```python
from build123d import *
from build123d.topology import SkipClean

# Parameters (mm, degrees)
SALIENTE_EXTRUIR3_DEPTH        = 342.9
SALIENTE_EXTRUIR3_DEPTH_BACK   = 342.9
CROQUIS3_R                     = 6.35
SALIENTE_EXTRUIR3_2_DEPTH      = 342.9
SALIENTE_EXTRUIR3_2_DEPTH_BACK = 342.9
CROQUIS4_W                     = 533.4
CROQUIS4_H                     = 165.1
SALIENTE_EXTRUIR4_DEPTH        = 555.498
VACIADO3_START                 = -265.43
VACIADO3_DEPTH                 = 530.86
VACIADO3_START_2               = -341.63
VACIADO3_2_OUTLINE_R           = 5.08
VACIADO3_2_DEPTH               = 683.26
REDONDEO5_R                    = 2.54
CROQUIS5_W                     = 152.4
CROQUIS5_H                     = 2.54
SALIENTE_EXTRUIR5_DEPTH        = 101.6
CORTAR_EXTRUIR2_DEPTH          = 676.270787465
CORTAR_EXTRUIR8_DEPTH          = 676.270787542


# Read off the part's stored shape, not the designer's step: Vaciado3
with BuildPart() as part:
    # Croquis3 → Saliente-Extruir3 (new, two sides: drawn at the far end of the back side and taken through both)
    with BuildSketch(Plane(origin=(0, 0, 0), x_dir=(0, 0, -1), z_dir=(1, 0, 0)).offset(-SALIENTE_EXTRUIR3_DEPTH_BACK)):
        Circle(CROQUIS3_R)
    extrude(amount=SALIENTE_EXTRUIR3_DEPTH + SALIENTE_EXTRUIR3_DEPTH_BACK)



with BuildPart() as body_2:
    # Croquis3 → Saliente-Extruir3 2 (new, two sides: drawn at the far end of the back side and taken through both)
    with BuildSketch(Plane(origin=(0, 0, 0), x_dir=(0, 0, -1), z_dir=(1, 0, 0)).offset(-SALIENTE_EXTRUIR3_2_DEPTH_BACK)):
        with Locations((165.1, 0)):
            Circle(CROQUIS3_R)
    extrude(amount=SALIENTE_EXTRUIR3_2_DEPTH + SALIENTE_EXTRUIR3_2_DEPTH_BACK)


with BuildPart() as part_1:
    add(part.part)

    add(body_2.part)  # Saliente-Extruir4 merges body 2
    # Croquis4 → Saliente-Extruir4 (add)
    with BuildSketch(Plane(origin=(0, 0, 0), x_dir=(1, 0, 0), z_dir=(0, 1, 0))):
        with Locations((0, 82.55)):
            Rectangle(CROQUIS4_W, CROQUIS4_H)
    extrude(amount=-SALIENTE_EXTRUIR4_DEPTH)

    # Vaciado3 outline → Vaciado3 (cut)
    with BuildSketch(Plane.YZ.offset(VACIADO3_START)):
        with BuildLine():
            Line((-554.228, -163.83), (-4.91868885, -163.83))
            ThreePointArc((-4.91868885, -163.83), (3.110851973, -169.116092628), (0, -160.02))
            Line((0, -160.02), (0, -5.08))
            ThreePointArc((0, -5.08), (3.110851973, 4.016092628), (-4.91868885, -1.27))
            Line((-4.91868885, -1.27), (-554.228, -1.27))
            Line((-554.228, -1.27), (-554.228, -163.83))
        make_face()
    extrude(amount=VACIADO3_DEPTH, mode=Mode.SUBTRACT)

    # Vaciado3 2 outline → Vaciado3 2 (cut)
    with BuildSketch(Plane.YZ.offset(VACIADO3_START_2)):
        with Locations((0, -165.1)):
            Circle(VACIADO3_2_OUTLINE_R)
        Circle(VACIADO3_2_OUTLINE_R)
    extrude(amount=VACIADO3_2_DEPTH, mode=Mode.SUBTRACT)

    # Redondeo5
    # the kernel refuses this fillet: 2.54 mm, written as the material it takes off along each edge
    with BuildSketch(Plane(origin=(-264.16, -552.958, -2.54), x_dir=(0, 0, 1), z_dir=(-1, 0, 0))) as redondeo5_piece_1_section:
        Polygon((0, 0), (REDONDEO5_R * 1.02, 0), (REDONDEO5_R * 1.02, -REDONDEO5_R * 1.02), (0, -REDONDEO5_R * 1.02), align=None)
    redondeo5_piece_1 = extrude(amount=REDONDEO5_R * 1.02, mode=Mode.PRIVATE)
    redondeo5_piece_1 = redondeo5_piece_1 - Plane(origin=(-264.16, -552.958, -2.54), x_dir=(0, 0.7071067811865475, -0.7071067811865475), z_dir=(-1, 0, 0)) * Sphere(REDONDEO5_R, mode=Mode.PRIVATE)
    add(redondeo5_piece_1, mode=Mode.SUBTRACT)
    with BuildSketch(Plane(origin=(-264.16, -552.958, -162.56), x_dir=(0, -1, 0), z_dir=(-1, 0, 0))) as redondeo5_piece_2_section:
        Polygon((0, 0), (REDONDEO5_R * 1.02, 0), (REDONDEO5_R * 1.02, -REDONDEO5_R * 1.02), (0, -REDONDEO5_R * 1.02), align=None)
    redondeo5_piece_2 = extrude(amount=REDONDEO5_R * 1.02, mode=Mode.PRIVATE)
    redondeo5_piece_2 = redondeo5_piece_2 - Plane(origin=(-264.16, -552.958, -162.56), x_dir=(0, 0.7071067811865475, 0.7071067811865475), z_dir=(-1, 0, 0)) * Sphere(REDONDEO5_R, mode=Mode.PRIVATE)
    add(redondeo5_piece_2, mode=Mode.SUBTRACT)
    with BuildSketch(Plane(origin=(264.16, -552.958, -2.54), x_dir=(1, 0, 0), z_dir=(0, 0, 1))) as redondeo5_piece_3_section:
        Polygon((0, 0), (REDONDEO5_R * 1.02, 0), (REDONDEO5_R * 1.02, -REDONDEO5_R * 1.02), (0, -REDONDEO5_R * 1.02), align=None)
    redondeo5_piece_3 = extrude(amount=REDONDEO5_R * 1.02, mode=Mode.PRIVATE)
    redondeo5_piece_3 = redondeo5_piece_3 - Plane(origin=(264.16, -552.958, -2.54), x_dir=(-0.7071067811865475, 0.7071067811865475, 0), z_dir=(0, 0, 1)) * Sphere(REDONDEO5_R, mode=Mode.PRIVATE)
    add(redondeo5_piece_3, mode=Mode.SUBTRACT)
    with BuildSketch(Plane(origin=(264.16, -552.958, -162.56), x_dir=(1, 0, 0), z_dir=(0, -1, 0))) as redondeo5_piece_4_section:
        Polygon((0, 0), (REDONDEO5_R * 1.02, 0), (REDONDEO5_R * 1.02, -REDONDEO5_R * 1.02), (0, -REDONDEO5_R * 1.02), align=None)
    redondeo5_piece_4 = extrude(amount=REDONDEO5_R * 1.02, mode=Mode.PRIVATE)
    redondeo5_piece_4 = redondeo5_piece_4 - Plane(origin=(264.16, -552.958, -162.56), x_dir=(-0.7071067811865474, 0, 0.7071067811865477), z_dir=(0, -1, 0)) * Sphere(REDONDEO5_R, mode=Mode.PRIVATE)
    add(redondeo5_piece_4, mode=Mode.SUBTRACT)
    with BuildSketch(Plane(origin=(266.7, 0, -164.249261314), x_dir=(0, -1, 0), z_dir=(0, 0, 1))) as redondeo5_piece_5_section:
        with BuildLine():
            CenterArc((2.199704526, -2.54), REDONDEO5_R, 90, 60)
            Line((0, -1.27), (0, 0))
            Line((0, 0), (2.199704526, 0))
        make_face()
    redondeo5_piece_5 = extrude(amount=163.398522628, mode=Mode.PRIVATE)
    redondeo5_piece_5 = redondeo5_piece_5 - Plane(origin=(266.364103935, 0, 0), x_dir=(0, 0, -1), z_dir=(-1, 0, 0)) * Cylinder(6.35, 336, mode=Mode.PRIVATE)
    redondeo5_piece_5 = redondeo5_piece_5 - Plane(origin=(266.364103935, 0, -165.1), x_dir=(0, 0, -1), z_dir=(-1, 0, 0)) * Cylinder(6.35, 336, mode=Mode.PRIVATE)
    add(redondeo5_piece_5, mode=Mode.SUBTRACT)
    with BuildSketch(Plane(origin=(-266.7, 0, -0.850738686), x_dir=(1, 0, 0), z_dir=(0, 0, -1))) as redondeo5_piece_6_section:
        with BuildLine():
            CenterArc((2.54, 2.199704526), REDONDEO5_R, 180, 60)
            Line((0, 2.199704526), (0, 0))
            Line((0, 0), (1.27, 0))
        make_face()
    redondeo5_piece_6 = extrude(amount=163.398522628, mode=Mode.PRIVATE)
    redondeo5_piece_6 = redondeo5_piece_6 - Plane(origin=(-266.364103935, 0, 0), x_dir=(0, 0, -1), z_dir=(-1, 0, 0)) * Cylinder(6.35, 336, mode=Mode.PRIVATE)
    redondeo5_piece_6 = redondeo5_piece_6 - Plane(origin=(-266.364103935, 0, -165.1), x_dir=(0, 0, -1), z_dir=(-1, 0, 0)) * Cylinder(6.35, 336, mode=Mode.PRIVATE)
    add(redondeo5_piece_6, mode=Mode.SUBTRACT)
    with BuildSketch(Plane(origin=(-266.7, 0, 0), x_dir=(1, 0, 0), z_dir=(0, -1, 0))) as redondeo5_piece_7_section:
        with BuildLine():
            CenterArc((REDONDEO5_R, -REDONDEO5_R), REDONDEO5_R, 90, 90)
            Line((0, -REDONDEO5_R), (0, 0))
            Line((0, 0), (REDONDEO5_R, 0))
        make_face()
    redondeo5_piece_7 = extrude(amount=552.958, mode=Mode.PRIVATE)
    redondeo5_piece_7 = redondeo5_piece_7 - Plane(origin=(-266.132673367, 0, 0), x_dir=(0, 0, -1), z_dir=(-1, 0, 0)) * Cylinder(6.35, 1117, mode=Mode.PRIVATE)
    add(redondeo5_piece_7, mode=Mode.SUBTRACT)
    with BuildSketch(Plane(origin=(-266.7, -555.498, -2.54), x_dir=(0, 1, 0), z_dir=(0, 0, -1)), Plane(origin=(266.7, -555.498, -162.56), x_dir=(0, 1, 0), z_dir=(0, 0, 1))) as redondeo5_piece_8:
        with BuildLine():
            CenterArc((REDONDEO5_R, REDONDEO5_R), REDONDEO5_R, 180, 90)
            Line((0, REDONDEO5_R), (0, 0))
            Line((0, 0), (REDONDEO5_R, 0))
        make_face()
    extrude(amount=160.02, mode=Mode.SUBTRACT)
    with BuildSketch(Plane(origin=(-266.7, 0, -165.1), x_dir=(0, 0, 1), z_dir=(0, -1, 0))) as redondeo5_piece_9_section:
        with BuildLine():
            CenterArc((REDONDEO5_R, -REDONDEO5_R), REDONDEO5_R, 90, 90)
            Line((0, -REDONDEO5_R), (0, 0))
            Line((0, 0), (REDONDEO5_R, 0))
        make_face()
    redondeo5_piece_9 = extrude(amount=552.958, mode=Mode.PRIVATE)
    redondeo5_piece_9 = redondeo5_piece_9 - Plane(origin=(-266.132672665, 0, -165.1), x_dir=(0, 0, -1), z_dir=(-1, 0, 0)) * Cylinder(6.35, 1117, mode=Mode.PRIVATE)
    add(redondeo5_piece_9, mode=Mode.SUBTRACT)
    with BuildSketch(Plane(origin=(266.7, 0, 0), x_dir=(-1, 0, 0), z_dir=(0, -1, 0))) as redondeo5_piece_10_section:
        with BuildLine():
            CenterArc((REDONDEO5_R, REDONDEO5_R), REDONDEO5_R, 180, 90)
            Line((0, REDONDEO5_R), (0, 0))
            Line((0, 0), (REDONDEO5_R, 0))
        make_face()
    redondeo5_piece_10 = extrude(amount=552.958, mode=Mode.PRIVATE)
    redondeo5_piece_10 = redondeo5_piece_10 - Plane(origin=(266.132673367, 0, 0), x_dir=(0, 0, -1), z_dir=(-1, 0, 0)) * Cylinder(6.35, 1117, mode=Mode.PRIVATE)
    add(redondeo5_piece_10, mode=Mode.SUBTRACT)
    with BuildSketch(Plane(origin=(264.16, -555.498, 0), x_dir=(0, 1, 0), z_dir=(-1, 0, 0))) as redondeo5_piece_11:
        with BuildLine():
            CenterArc((REDONDEO5_R, REDONDEO5_R), REDONDEO5_R, 180, 90)
            Line((0, REDONDEO5_R), (0, 0))
            Line((0, 0), (REDONDEO5_R, 0))
        make_face()
    extrude(amount=528.32, mode=Mode.SUBTRACT)
    with BuildSketch(Plane(origin=(-264.16, -555.498, -165.1), x_dir=(0, 0, 1), z_dir=(1, 0, 0))) as redondeo5_piece_12:
        with BuildLine():
            CenterArc((REDONDEO5_R, -REDONDEO5_R), REDONDEO5_R, 90, 90)
            Line((0, -REDONDEO5_R), (0, 0))
            Line((0, 0), (REDONDEO5_R, 0))
        make_face()
    extrude(amount=528.32, mode=Mode.SUBTRACT)
    with BuildSketch(Plane(origin=(266.7, 0, -165.1), x_dir=(0, 0, 1), z_dir=(0, -1, 0))) as redondeo5_piece_13_section:
        with BuildLine():
            CenterArc((REDONDEO5_R, REDONDEO5_R), REDONDEO5_R, 180, 90)
            Line((0, REDONDEO5_R), (0, 0))
            Line((0, 0), (REDONDEO5_R, 0))
        make_face()
    redondeo5_piece_13 = extrude(amount=552.958, mode=Mode.PRIVATE)
    redondeo5_piece_13 = redondeo5_piece_13 - Plane(origin=(266.132672665, 0, -165.1), x_dir=(0, 0, -1), z_dir=(-1, 0, 0)) * Cylinder(6.35, 1117, mode=Mode.PRIVATE)
    add(redondeo5_piece_13, mode=Mode.SUBTRACT)

    # Croquis5 → Saliente-Extruir5 (add)
    with SkipClean():  # the faces are left unmerged after this step: merging them gives an invalid solid
        with BuildSketch(Plane(origin=(0, 0, 0), x_dir=(1, 0, 0), z_dir=(0, 1, 0))):
            with Locations((0, 164.974335694)):
                Rectangle(CROQUIS5_W, CROQUIS5_H)
            Rectangle(CROQUIS5_W, CROQUIS5_H)
        extrude(amount=SALIENTE_EXTRUIR5_DEPTH)

    # Croquis6 → Cortar-Extruir2 (cut, through all)
    with SkipClean():  # the faces are left unmerged after this step: merging them gives an invalid solid
        with BuildSketch(Plane.XY.offset(1.27)):
            with BuildLine():
                Line((-50.8, 6.221703947), (50.8, 6.221703947))
                ThreePointArc((50.8, 6.221703947), (0, 57.021703947), (-50.8, 6.221703947))
            make_face()
        extrude(amount=-CORTAR_EXTRUIR2_DEPTH, mode=Mode.SUBTRACT)

    # Croquis7 → Cortar-Extruir8 (cut, through all)
    with SkipClean():  # the faces are left unmerged after this step: merging them gives an invalid solid
        with BuildSketch(Plane.XY.offset(1.27)):
            with BuildLine():
                Line((-71.12, 6.221703947), (-76.2, 6.221703947))
                Line((-76.2, 6.221703947), (-76.2, 101.6))
                Line((-76.2, 101.6), (76.2, 101.6))
                Line((76.2, 101.6), (76.2, 6.221703947))
                Line((76.2, 6.221703947), (71.12, 6.221703947))
                ThreePointArc((71.12, 6.221703947), (0, 77.341703947), (-71.12, 6.221703947))
            make_face()
        extrude(amount=-CORTAR_EXTRUIR8_DEPTH, mode=Mode.SUBTRACT)


solid = part_1.part
```
Verification items for the finished model (mm, model axes). A direction names the side the tool comes from. Give positions to 0.01 mm unless a question says otherwise; leave off trailing zeros. Order: outer loops, then holes, each group sorted by start corner. A loop starts at its lowest first (then second) coordinate and runs counter-clockwise, first axis right, second up. Notation, with made-up numbers: (21, 54.25) -> (44, 54.25) arc R21 cw to (44, 64.25) -> close; hole circle Ø7 at (53.5, 64). An arc over 180 degrees is marked (long way). Use a Markdown table: item, result.
1) Mould release check, pull along X, two halves, no side actions. Record for faces 6 (the flat face through (-4, -283, -163.83)), 7 (the flat face through (-266.7, -274, -81)), 8 (the flat face through (-17, 57, 1.27)): pulls with the +X half, pulls with the -X half, needs draft (parallel to the pull), parting line crosses it, or undercut.
Results:
| item | result |
|---|---|
| face 6 | undercut |
| face 7 | pulls with the -X half |
| face 8 | needs draft |
2) Section check D-D, the plane x = 166.5. Record the boundary of the cut face in (y, z).
Results:
| item | result |
|---|---|
| outline | (-555.5, -162.56) arc R2.54 ccw to (-552.96, -165.1) -> (-6.35, -165.1) arc R6.35 ccw (long way) to (0, -158.75) -> (0, -160.02) arc R5.08 cw (long way) to (-4.92, -163.83) -> (-554.23, -163.83) -> (-554.23, -1.27) -> (-4.92, -1.27) arc R5.08 cw (long way) to (0, -5.08) -> (0, -6.35) arc R6.35 ccw (long way) to (-6.35, 0) -> (-552.96, 0) arc R2.54 ccw to (-555.5, -2.54) -> close |
3) Material ranges on probe 1 along X at (y, z) = (-208.5, -91); probe 2 along Z at (x, y) = (-132.5, -196.5); probe 3 along Y at (x, z) = (-156.5, -41), recorded low to high.
Results:
| item | result |
|---|---|
| probe 1 | -266.7 to -265.43, 265.43 to 266.7 |
| probe 2 | -165.1 to -163.83, -1.27 to 0 |
| probe 3 | -555.5 to -554.23 |
4) Tool access check on faces 1 (the flat face through (-17, 57, -1.27)), 2 (the cylindrical face through (1.12, 57.01, -165.02)), 3 (the flat face through (-4, -276, 0)), 4 (the flat face through (-17, 57, -166.244)), 5 (the flat face through (-4, -276, -165.1)). Record the directions out of +Z, -Z, +X, -X, +Y, -Y that give a thin tool (end or side, any length) a straight path to the whole face; none if there is none.
Results:
| item | result |
|---|---|
| face 1 | +X, -X, +Y |
| face 2 | +Z, -Z |
| face 3 | +Z, +X, -X, -Y |
| face 4 | -Z, +X, -X, +Y |
| face 5 | -Z, +X, -X, -Y |
5) Section check C-C, the plane y = 19. Record the boundary of the cut face in (x, z), then the cut area to 3 significant figures.
Results:
| item | result |
|---|---|
| outline | (-69.96, -166.24) -> (-49.17, -166.24) -> (-49.17, -163.7) -> (-69.96, -163.7) -> close; (-69.96, -1.27) -> (-49.17, -1.27) -> (-49.17, 1.27) -> (-69.96, 1.27) -> close; (49.17, -166.24) -> (69.96, -166.24) -> (69.96, -163.7) -> (49.17, -163.7) -> close; (49.17, -1.27) -> (69.96, -1.27) -> (69.96, 1.27) -> (49.17, 1.27) -> close |
| area | 211 mm² |
6) Depth check by flat-ended pin: pin 1 Ø1.3 at (x, z) = (17.5, 0) entering from -Y; pin 2 Ø5 at (x, y) = (112.5, -348.5) entering from +Z; pin 3 Ø1.5 at (x, y) = (37.5, 3) entering from +Z; pin 4 Ø5.5 at (x, y) = (-32.5, 1.5) entering from -Z. Enter the tip coordinate at first touch or a pass-through.
Results:
| item | result |
|---|---|
| pin 1 | y = -554.65 |
| pin 2 | z = 0 |
| pin 3 | z = 5.94 |
| pin 4 | z = -171.45 |
7) Section check B-B, the plane y = -428. Record the boundary of the cut face in (x, z).
Results:
| item | result |
|---|---|
| outline | (-266.7, -162.56) arc R2.54 ccw to (-264.16, -165.1) -> (264.16, -165.1) arc R2.54 ccw to (266.7, -162.56) -> (266.7, -2.54) arc R2.54 ccw to (264.16, 0) -> (-264.16, 0) arc R2.54 ccw to (-266.7, -2.54) -> close; hole (-265.43, -163.83) -> (265.43, -163.83) -> (265.43, -1.27) -> (-265.43, -1.27) -> close |
8) Section check A-A, the plane x = 301. Record the boundary of the cut face in (y, z), then the cut area to 3 significant figures.
Results:
| item | result |
|---|---|
| outline | circle Ø12.7 at (0, -165.1); circle Ø12.7 at (0, 0); hole circle Ø10.16 at (0, -165.1); hole circle Ø10.16 at (0, 0) |
| area | 91.2 mm² |
